Check sheet for the drawn part. Datum: minimum x, y, z corner. Units: mm. Give positions to 0.01 mm unless a question says otherwise; leave off trailing zeros. Write each loop counter-clockwise with the first axis right and the second up, starting at its lowest first coordinate (ties: lowest second). Pieces come first, ordered by that corner, then holes. Notation, with made-up numbers: (30, 67) - (71, 67) arc R26 cw to (71, 102) - close; hole circle Ø5 at (47, 40). An arc over 180 degrees is marked (long way). Use a Markdown table: item, result.
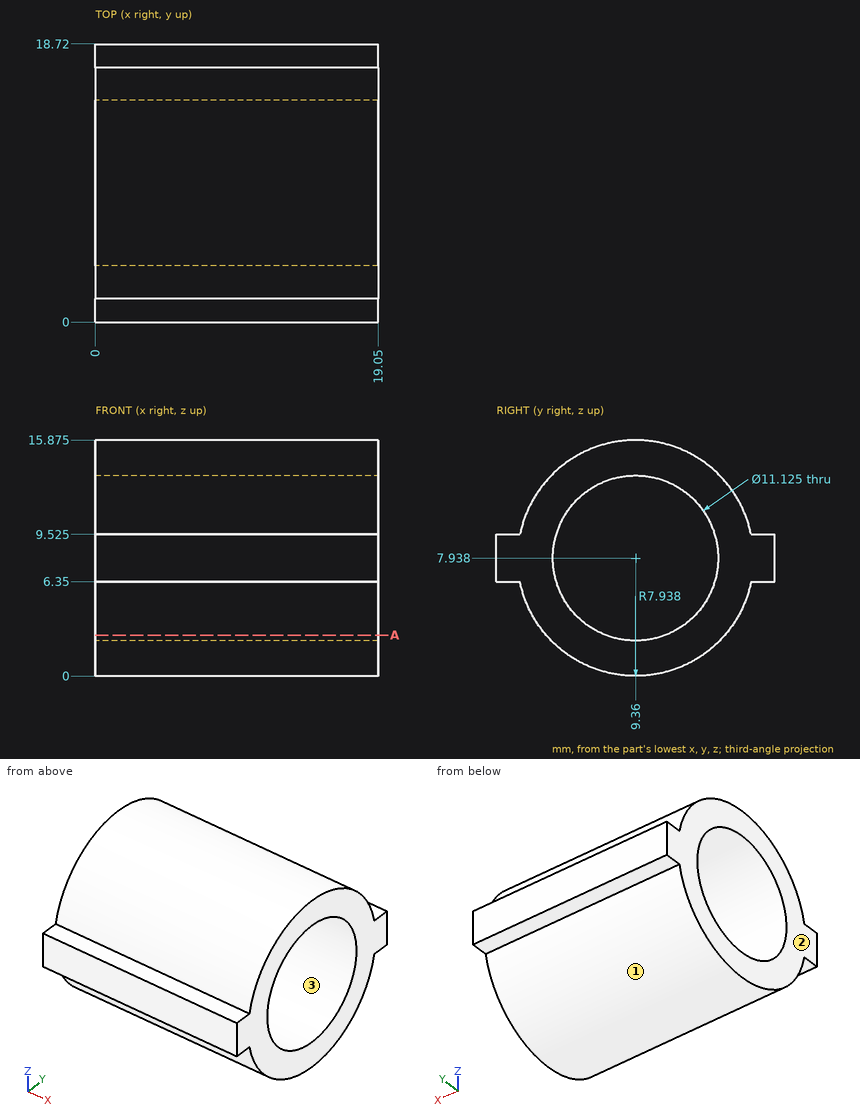
1) Section check A-A on z = 2.75. Record the boundary of the cut face in (x, y), then the cut area to 3 significant figures.
Working result:
| item | result |
|---|---|
| outline | (0, 3.35) - (19.05, 3.35) - (19.05, 7.35) - (0, 7.35) - close; (0, 11.37) - (19.05, 11.37) - (19.05, 15.37) - (0, 15.37) - close |
| area | 152 mm² |
2) Depth check by flat-ended pin: P1, Ø4, axis at x = 13, z = 14, coming from the +Y side; P2, Ø6.5, axis at y = 9.36, z = 7.94, coming from the -X side; P3, Ø1.5, axis at x = 3.5, y = 5.5, coming from the -Z side (1 decimal); P4, Ø0.5, axis at x = 11, y = 1, coming from the +Z side (1 decimal). Enter the tip coordinate at first touch or a pass-through.
Working result:
| item | result |
|---|---|
| P1 | stops at y = 16.18 |
| P2 | passes through |
| P3 | stops at z = 0.6 |
| P4 | stops at z = 9.5 |
3) Mould release check, pull along Y, two halves, no side actions. Record for the marked faces 1, 2 and 3: pulls with the +Y half, pulls with the -Y half, needs draft (parallel to the pull), parting line crosses it, or undercut.
Working result:
| item | result |
|---|---|
| face 1 | parting line crosses it |
| face 2 | needs draft |
| face 3 | undercut |
4) Material ranges on L1, parallel to Z at x = 12, y = 9.5; L2, parallel to Y at x = 6.5, z = 4.75; L3, parallel to Z at x = 16, y = 11.75 (1 decimal), recorded low to high. Write a range as from..to.
Working result:
| item | result |
|---|---|
| L1 | z = 0..2.38, 13.5..15.87 |
| L2 | y = 2.09..4.8, 13.92..16.63 |
| L3 | z = 0.4..2.9, 13..15.5 |
